Design review of the part built by this model. Coordinates are the model's own, in mm. Face numbers are marked on the shaded views. Coordinates: 2 decimals unless noted, no trailing zeros. Loops run counter-clockwise (first coordinate to the right, second up) from the corner with the lowest first, then second, coordinate; pieces in that order, holes last.
Q1. Add section B-B on y = -1.05. Give the boundary of the cut face in (x, z) (3 decimals).
Q2. Wall thickness on probe 1 along X at (y, z) = (-2.4, 3.15); probe 2 along X at (y, z) = (-4.2, 4.5); probe 3 along Y at (x, z) = (34, 1.45): over which ranges is each line inside the solid? List them lowest first.
Q3. Draft analysis for pull direction Z (two halves, no side actions). For the marked faces 1, 2, 3 and 4, state which applies: released by +Z, released by -Z, zero draft, split by the parting line, or undercut.
Q4. Add section A-A on z = 3.7. Give the boundary of the cut face in (x, y).
Q5. For P1, Ø0.8, axis at x = 1, y = -2.5, coming from the -Z side; P2, Ø1.5, axis at y = -2, z = 1.5, coming from the +X side; P3, Ø2, axis at y = -3, z = 1.5, coming from the -X side; P4, Ø1.5, axis at y = -1, z = 1, coming from the -X side, all flat-tipped, find the tip position at first contact; note any pin that passes through.
Q6. Add section C-C on y = -3.8. Give the boundary of the cut face in (x, z) (3 decimals).
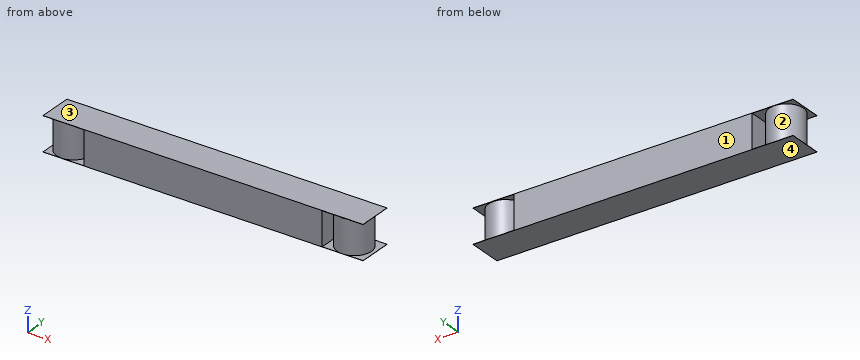
```python
from build123d import *

# Parameters (mm, degrees)
SKETCH1_W           = 47
SKETCH1_H           = 5
BOSS_EXTRUDE1_DEPTH = 5
SKETCH3_W           = 6
SKETCH3_H           = 5.264109691
SKETCH3_H_2         = 5.408392742
CUT_EXTRUDE1_DEPTH  = 2.475
SKETCH4_R           = 2.5
BOSS_EXTRUDE2_DEPTH = 4.95
SKETCH5_R           = 2.5
BOSS_EXTRUDE3_DEPTH = 4.95


with BuildPart() as part:
    # Sketch1 → Boss-Extrude1 (new body)
    with BuildSketch(Plane.XY):
        with Locations((23.5, -2.5)):
            Rectangle(SKETCH1_W, SKETCH1_H)
    extrude(amount=BOSS_EXTRUDE1_DEPTH)

    # Sketch3 → Cut-Extrude1 (cut, symmetric)
    with BuildSketch(Plane.XY.offset(2.5)):
        with Locations((3, -2.632054846)):
            Rectangle(SKETCH3_W, SKETCH3_H)
        with Locations((44, -2.55991332)):
            Rectangle(SKETCH3_W, SKETCH3_H_2)
    extrude(amount=CUT_EXTRUDE1_DEPTH, both=True, mode=Mode.SUBTRACT)

    # Sketch4 → Boss-Extrude2 (add)
    with BuildSketch(Plane.XY.offset(0.025)):
        with Locations(Location((44, -2.555494601, 0), (0, 0, 257.905173383))):
            Circle(SKETCH4_R)
    extrude(amount=BOSS_EXTRUDE2_DEPTH)

    # Sketch5 → Boss-Extrude3 (add)
    with BuildSketch(Plane.XY.offset(0.025)):
        with Locations(Location((2.73169256, -2.5, 0), (0, 0, 90))):
            Circle(SKETCH5_R)
    extrude(amount=BOSS_EXTRUDE3_DEPTH)


solid = part.part
```
Entries:
1. outline: (0, 0) - (47, 0) - (47, 0.025) - (45.996, 0.025) - (45.996, 4.975) - (47, 4.975) - (47, 5) - (0, 5) - (0, 4.975) - (0.695, 4.975) - (0.695, 0.025) - (0, 0.025) - close; hole (4.768, 0.025) - (6, 0.025) - (6, 4.975) - (4.768, 4.975) - close; hole (41, 0.025) - (42.004, 0.025) - (42.004, 4.975) - (41, 4.975) - close
2. probe 1: x = 0.23 to 5.23, 6 to 41, 41.5 to 46.5
2. probe 2: x = 0.9 to 4.56, 6 to 41, 42.12 to 45.88
2. probe 3: y = -5 to 0
3. face 1: zero draft
3. face 2: undercut
3. face 3: released by +Z
3. face 4: released by -Z
4. outline: circle Ø5 at (2.73, -2.5); (6, -5) - (41, -5) - (41, 0) - (6, 0) - close; circle Ø5 at (44, -2.56)
5. P1: stops at z = 0
5. P2: stops at x = 46.5
5. P3: stops at x = 0.23
5. P4: stops at x = 0.35
6. outline: (0, 0) - (47, 0) - (47, 0.025) - (46.168, 0.025) - (46.168, 4.975) - (47, 4.975) - (47, 5) - (0, 5) - (0, 4.975) - (0.596, 4.975) - (0.596, 0.025) - (0, 0.025) - close; hole (4.867, 0.025) - (6, 0.025) - (6, 4.975) - (4.867, 4.975) - close; hole (41, 0.025) - (41.832, 0.025) - (41.832, 4.975) - (41, 4.975) - close
